Model file for the job. Use its own axes, mm. Face numbers are marked on the shaded views. Round coordinates to 2 decimals unless told otherwise and drop trailing zeros. Order: outer loops, then holes, each group sorted by start corner. A loop starts at its lowest first (then second) coordinate and runs counter-clockwise, first axis right, second up. Notation, with made-up numbers: M 54.25,37.5 L 79.25,37.5 A15 cw 79.25,44.5 Z; hole C -11.5,64 d4. An arc over 180 degrees is marked long. Return JSON: item names as keys, results as strings. Group by question number.
Item 1: Slice it at A-A on x = 103. Write the cut outline in (y, z) (3 decimals), then the cut area to 3 significant figures.
Item 2: Slice it at D-D on z = 56.5. Write the cut outline in (x, y) (3 decimals), then the cut area to 3 significant figures.
Item 3: Slice it at B-B on z = 0. Write the cut outline in (x, y) (3 decimals).
Item 4: Probe line 1 along X through (y, z) = (-20.5, -100) (3 decimals); line 2 along Z through (x, y) = (211.5, -37) (3 decimals); line 3 along Y through (x, z) = (125, -147.5). List the from-to ranges inside material, lowest first.
Item 5: Slice it at C-C on y = -45.5. Write the cut outline in (x, z) (3 decimals), then the cut area to 3 significant figures.
Item 6: Pull direction Z, two halves, no side cores. Call the marked faces 1 and 2: pulls with the +Z half, pulls with the -Z half, needs draft (parallel to the pull), parting line crosses it, or undercut.
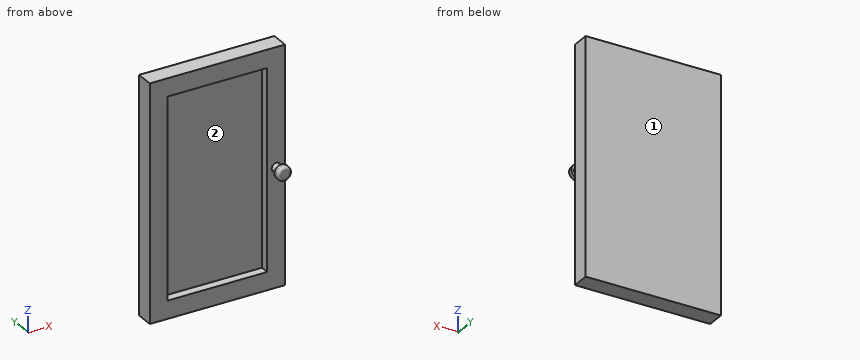
from build123d import *

# Parameters (mm, degrees)
F0_W     = 288.925
F0_H     = 501.65
F1_DEPTH = 19.05
F2_W     = 288.925
F2_H     = 501.65
F2_W_2   = 212.725
F2_H_2   = 425.45
F3_DEPTH = 19.05


with BuildPart() as f1:
    # F0 (on Front) → F1 (new body)
    with BuildSketch(Plane.XZ):
        with Locations((144.4625, 0)):
            Rectangle(F0_W, F0_H)
    extrude(amount=F1_DEPTH)

    # F2 (on face) → F3 (join)
    with BuildSketch(Plane.XZ.offset(19.05)):
        with Locations((144.4625, 0)):
            Rectangle(F2_W, F2_H)
        with Locations((144.4625, 0)):
            Rectangle(F2_W_2, F2_H_2, mode=Mode.SUBTRACT)
    extrude(amount=F3_DEPTH)

    # F4 (on Top) → F5 (revolve)
    with BuildSketch(Plane.XY):
        with BuildLine():
            Line((279.4, -57.15), (279.4, 0))
            Line((279.4, 0), (269.875, 0))
            Line((269.875, 0), (269.875, -69.85))
            Line((269.875, -69.85), (278.765, -69.85))
            ThreePointArc((278.765, -69.85), (283.255128, -67.990128), (285.115, -63.5))
            Line((285.115, -63.5), (285.115, -57.15))
            Line((285.115, -57.15), (279.4, -57.15))
        make_face()
    revolve(axis=Axis((269.875, -127, 0), (0, -1, 0)))


solid = f1.part
Output values:
{
 "1": {"outline": "M -38.1,-250.825 L 0,-250.825 L 0,250.825 L -38.1,250.825 L -38.1,212.725 L -19.05,212.725 L -19.05,-212.725 L -38.1,-212.725 Z", "area": "11,000 mm²"},
 "2": {"outline": "M 0,-38.1 L 38.1,-38.1 L 38.1,-19.05 L 250.825,-19.05 L 250.825,-38.1 L 288.925,-38.1 L 288.925,0 L 0,0 Z", "area": "6,960 mm²"},
 "3": {"outline": "M 0,-38.1 L 38.1,-38.1 L 38.1,-19.05 L 250.825,-19.05 L 250.825,-38.1 L 260.35,-38.1 L 260.35,-57.15 L 254.635,-57.15 L 254.635,-63.5 A6.35 ccw 260.985,-69.85 L 278.765,-69.85 A6.35 ccw 285.115,-63.5 L 285.115,-57.15 L 279.4,-57.15 L 279.4,-38.1 L 288.925,-38.1 L 288.925,0 L 0,0 Z"},
 "4": {"line 1": "0 to 38.1, 250.825 to 288.925", "line 2": "-250.825 to -212.725, 212.725 to 250.825", "line 3": "-19.05 to 0"},
 "5": {"outline": "C 269.875,0 d19.05", "area": "285 mm²"},
 "6": {"face 1": "needs draft", "face 2": "undercut"}
}
